Part model, mm, in its own coordinate system. Face numbers are marked on the shaded views. A direction names the side the tool comes from. Round coordinates to 2 decimals unless told otherwise and drop trailing zeros. Order: outer loops, then holes, each group sorted by start corner. A loop starts at its lowest first (then second) coordinate and runs counter-clockwise, first axis right, second up. Notation, with made-up numbers: (-36, 50) - (18, 50) arc R26 cw to (18, 70) - close; hole circle Ø9 at (-3, 36). An arc over 180 degrees is marked (long way). Return JSON: item names as keys, results as strings. Group by question number.
Item 1: Drop flat-ended pins along their axis: pin 1 (1.5 mm diameter, centred on x = 42.5, z = -4, fed in from -Y); pin 2 (2 mm diameter, centred on y = 35.5, z = 2.5, fed in from -X); pin 3 (2 mm diameter, centred on x = -161, z = 55, fed in from +Y). Give the stop position or say it passes through.
Item 2: Tool access for the marked faces 1, 2, 3, 4 and 5: list every direction of +Z, -Z, +X, -X, +Y, -Y with a clear straight run to the whole face (end or side of a thin tool).
Item 3: Probe probe 1 along X at (y, z) = (-97.5, 2.5); probe 2 along Y at (x, z) = (141.5, -118); probe 3 along Z at (x, y) = (294, 130) (3 decimals). List the from-to ranges inside material, lowest first.
Item 4: Saw through at B-B on z = 56.5. List the corners of the cut face in (x, y), and give its area (3 significant figures).
Item 5: Saw through at C-C on x = 275. List the corners of the cut face in (y, z) (3 decimals), and give its area (3 significant figures).
```python
from build123d import *

# Parameters (mm, degrees)
F1_DEPTH      = 334.9625
F1_DEPTH_BACK = 334.9625
F2_W          = 100.0125
F2_H          = 431.8
F3_DEPTH      = 244.475


# Not quite as in the source:
# - a length typed as a fraction of an inch, garbled in the dataset ("3 / 203.2 mm" for 3/8 in), is restored


with BuildPart() as f1:
    # F0 (on Right) → F1 (new body, two sides)
    with BuildSketch(Plane.YZ) as f1_sk:
        Polygon((219.075, 127), (-219.075, 127), (-219.075, 92.075), (-215.9, 92.075), (-215.9, -152.4), (215.9, -152.4), (215.9, 92.075), (219.075, 92.075), align=None)
    extrude(amount=F1_DEPTH)
    extrude(f1_sk.sketch, amount=-F1_DEPTH_BACK)

    # F2 (on face) → F3 (cut, through all)
    with BuildSketch(Plane(origin=(0, 0, -152.4), x_dir=(1, 0, 0), z_dir=(0, 0, -1))):
        with Locations((-284.95625, 0)):
            Rectangle(F2_W, F2_H)
        with Locations((284.95625, 0)):
            Rectangle(F2_W, F2_H)
    extrude(amount=-F3_DEPTH, mode=Mode.SUBTRACT)


solid = f1.part
```
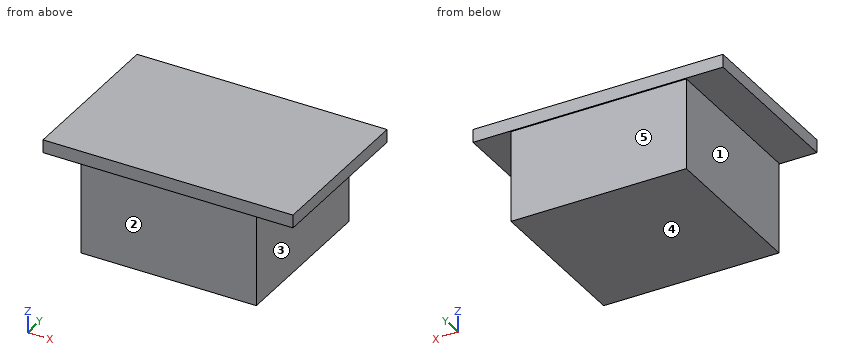
Filled in:
{
 "1": {"pin 1": "stops at y = -215.9", "pin 2": "stops at x = -234.95", "pin 3": "stops at y = 215.9"},
 "2": {"face 1": "-Z, -X, +Y, -Y", "face 2": "-Z, +X, -X, -Y", "face 3": "-Z, +X, +Y, -Y", "face 4": "-Z, +X, -X, +Y, -Y", "face 5": "-Z, +X, -X, +Y"},
 "3": {"probe 1": "x = -234.95 to 234.95", "probe 2": "y = -215.9 to 215.9", "probe 3": "z = 92.075 to 127"},
 "4": {"outline": "(-234.95, -215.9) - (234.95, -215.9) - (234.95, 215.9) - (-234.95, 215.9) - close", "area": "203,000 mm^2"},
 "5": {"outline": "(-219.075, 92.075) - (219.075, 92.075) - (219.075, 127) - (-219.075, 127) - close", "area": "15,300 mm^2"}
}
